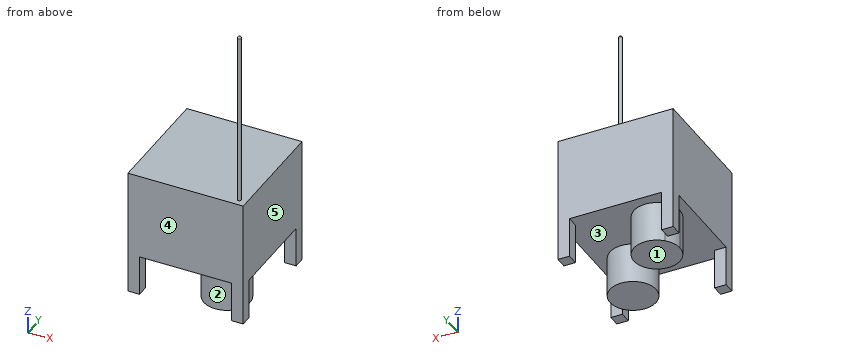
```python
from build123d import *

# Parameters (mm, degrees)
SKETCH1_W           = 100
SKETCH1_H           = 100
BOSS_EXTRUDE1_DEPTH = 110
SKETCH2_R           = 1.5875
BOSS_EXTRUDE2_DEPTH = 152.4
FILLET1_R           = 1.5875
SKETCH4_W           = 10
SKETCH4_H           = 80
SKETCH4_W_2         = 80
SKETCH4_H_2         = 10
CUT_EXTRUDE2_DEPTH  = 35
SKETCH5_R           = 20
BOSS_EXTRUDE3_DEPTH = 35


with BuildPart() as part:
    # Sketch1 → Boss-Extrude1 (new body)
    with BuildSketch(Plane.XY):
        Rectangle(SKETCH1_W, SKETCH1_H)
    extrude(amount=BOSS_EXTRUDE1_DEPTH)

    # Sketch2 → Boss-Extrude2 (add)
    with BuildSketch(Plane.XY.offset(110)):
        with Locations(Location((43.298646859, -43.309895232, 0), (0, 0, 180))):
            Circle(SKETCH2_R)
    extrude(amount=BOSS_EXTRUDE2_DEPTH)

    # Fillet1
    fillet1_edges = [part.edges().sort_by_distance(p)[0] for p in [
        (44.886146859, -43.309895232, 262.4),
    ]]
    fillet(fillet1_edges, radius=FILLET1_R)

    # Sketch4 → Cut-Extrude2 (cut)
    with BuildSketch(Plane(origin=(0, 0, 0), x_dir=(-1, 0, 0), z_dir=(0, 0, -1))):
        with Locations((45, 0)):
            Rectangle(SKETCH4_W, SKETCH4_H)
        Rectangle(SKETCH4_W_2, SKETCH4_H)
        with Locations((-45, 0)):
            Rectangle(SKETCH4_W, SKETCH4_H)
        with Locations((0, -45)):
            Rectangle(SKETCH4_W_2, SKETCH4_H_2)
        with Locations((0, 45)):
            Rectangle(SKETCH4_W_2, SKETCH4_H_2)
    extrude(amount=-CUT_EXTRUDE2_DEPTH, mode=Mode.SUBTRACT)

    # Sketch5 → Boss-Extrude3 (add)
    with BuildSketch(Plane(origin=(0, 0, 35), x_dir=(-1, 0, 0), z_dir=(0, 0, -1))):
        with BuildLine():
            ThreePointArc((35.355339059, 35.355339059), (7.071067812, 35.355339059), (7.071067812, 7.071067812))
            Line((7.071067812, 7.071067812), (35.355339059, 35.355339059))
        make_face()
        with BuildLine():
            Line((35.355339059, 35.355339059), (7.071067812, 7.071067812))
            ThreePointArc((7.071067812, 7.071067812), (28.866872083, 2.735612785), (41.213203436, 21.213203436))
            ThreePointArc((41.213203436, 21.213203436), (39.690794086, 28.866872083), (35.355339059, 35.355339059))
        make_face()
        with Locations((-21.213203436, -21.213203436)):
            Circle(SKETCH5_R)
    extrude(amount=BOSS_EXTRUDE3_DEPTH)


solid = part.part
```
Can you work these out from the model? Positions are in its coordinate system, mm. Face numbers are marked on the shaded views. A direction names the side the tool comes from. Round coordinates to 2 decimals unless told otherwise and drop trailing zeros. Loops run counter-clockwise (first coordinate to the right, second up) from the corner with the lowest first, then second, coordinate; pieces in that order, holes last. Notation, with made-up numbers: (-34, 47) -> (-21, 47) arc R6 ccw to (-21, 57) -> close; hole circle Ø2 at (54, 88.25). An arc over 180 degrees is marked (long way). One line per item, written item: value. Start each with the question number.
1. For pin 1 (10 mm diameter, centred on x = 7, y = -30, fed in from +Z); pin 2 (4 mm diameter, centred on x = 16, y = 29.5, fed in from -Z), each with a flat end and sliding along its axis, tell me the tip position at first contact or that it passes through.
2. For the marked faces 1 and 2, which set-ups out of +Z, -Z, +X, -X, +Y, -Y let a thin tool reach every point of the face, with its end or its side?
3. If we section it at B-B, the plane x = 30: Write out the boundary of the cut face in (y, z), then the cut area to 3 significant figures.
4. If we mould it in two halves opening along X, with no side actions, what happens to the marked faces 3, 4 and 5? For each: pulls with the +X half, pulls with the -X half, needs draft (parallel to the pull), parting line crosses it, or undercut.
5. If we section it at A-A, the plane z = 31.5: Write out the boundary of the cut face in (x, y), then the cut area to 3 significant figures.
6. If I drill on probe 1 along Z at (x, y) = (-28, 45.5); probe 2 along Y at (x, z) = (-44.5, 21.5); probe 3 along Z at (x, y) = (-30, 28.5), over which ranges is the centre line in solid material (lowest first)?
7. If we section it at C-C, the plane y = -26.5: Write out the boundary of the cut face in (x, z), then the cut area to 3 significant figures.
8. If we section it at D-D, the plane z = 213: Write out the boundary of the cut face in (x, y) (1 decimal).
Calculated:
1. pin 1: stops at z = 110
1. pin 2: stops at z = 35
2. face 1: -Z, +X, -X, +Y, -Y
2. face 2: -Z
3. outline: (-50, 35) -> (-39.18, 35) -> (-39.18, 0) -> (-3.25, 0) -> (-3.25, 35) -> (50, 35) -> (50, 110) -> (-50, 110) -> close
3. area: 8,760 mm²
4. face 3: undercut
4. face 4: needs draft
4. face 5: pulls with the +X half
5. outline: (-50, -50) -> (-40, -50) -> (-40, -40) -> (-50, -40) -> close; (-50, 40) -> (-40, 40) -> (-40, 50) -> (-50, 50) -> close; circle Ø40 at (-21.21, 21.21); circle Ø40 at (21.21, -21.21); (40, -50) -> (50, -50) -> (50, -40) -> (40, -40) -> close; (40, 40) -> (50, 40) -> (50, 50) -> (40, 50) -> close
5. area: 2,910 mm²
6. probe 1: z = 35 to 110
6. probe 2: y = -50 to -40, 40 to 50
6. probe 3: z = 0 to 110
7. outline: (-50, 35) -> (1.92, 35) -> (1.92, 0) -> (40.5, 0) -> (40.5, 35) -> (50, 35) -> (50, 110) -> (-50, 110) -> close
7. area: 8,850 mm²
8. outline: circle Ø3.2 at (43.3, -43.3)
